Geometry check sheet. Reference: the model listing, model coordinates, mm. Face numbers are marked on the shaded views. Give positions to 0.01 mm unless a question says otherwise; leave off trailing zeros. Write each loop counter-clockwise with the first axis right and the second up, starting at its lowest first coordinate (ties: lowest second). Pieces come first, ordered by that corner, then holes. Notation, with made-up numbers: (72, 9) - (121, 9) arc R28 cw to (121, 40) - close; hole circle Ø7 at (59, 43). An arc over 180 degrees is marked (long way). One line per question, with ' | ' between items. Start each with the question number.
Q1. Section check A-A on x = -7.75. Record the boundary of the cut face in (y, z).
Q2. Thickness scan on L1, parallel to X at y = -0.35, z = 0.55; L2, parallel to X at y = 0.05, z = 0.85; L3, parallel to Y at x = -6.75, z = 0.8. Record the ranges inside material, lowest first. Write a range as [from, to].
Q3. Section check B-B on y = -2.25. Record the boundary of the cut face in (x, z).
Q4. Section check D-D on y = 0.6. Record the boundary of the cut face in (x, z).
Q5. Release check for a two-part mould opening along X. For the marked faces 1 and 2 record: +X half, -X half, draft (parallel to the pull), parting line (faces both ways), or undercut.
Q6. Section check C-C on z = 0.85. Record the boundary of the cut face in (x, y) (1 decimal), and give its area (3 significant figures).
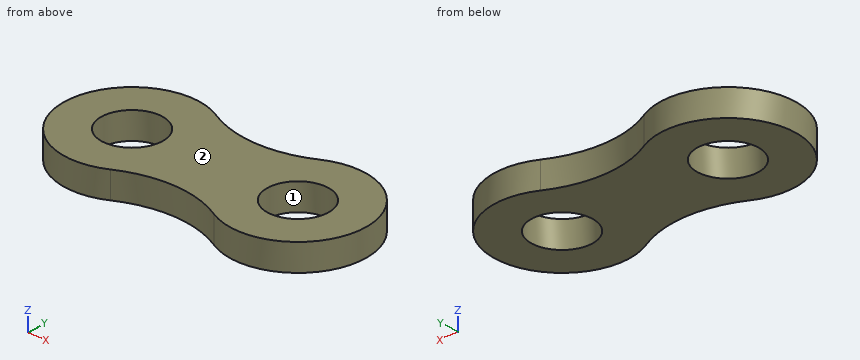
Autodesk Inventor part; units mm, degrees
ref_plane "YZ Plane" through (0, 0, 0) normal (1, 0, 0) x (0, 1, 0)
ref_plane "XZ Plane" through (0, 0, 0) normal (0, 1, 0) x (-1, 0, 0)
ref_plane "XY Plane" through (0, 0, 0) normal (0, 0, 1) x (1, 0, 0)
sketch "Sketch1" plane through (0, 0, 0) normal (0, 0, 1) x (1, 0, 0)
  arc A0 (-11.9712, 1.9221) -> (-8.0178, 1.9221) centre (-9.9945, 5.5697) ccw
  arc A1 (-8.0178, -2.5002) -> (-8.0178, 1.9221) centre (-6.8195, -0.289) ccw
  arc A2 (-8.0178, -2.5002) -> (-11.9712, -2.5002) centre (-9.9945, -6.1478) ccw
  arc A3 (-11.9712, 1.9221) -> (-11.9712, -2.5002) centre (-13.1695, -0.289) ccw
  circle A4 centre (-13.1695, -0.289) radius 1.135
  circle A5 centre (-6.8195, -0.289) radius 1.135
  point P0 (0, 0)
extrude "Extrusion1" add sketch "Sketch1" along normal blind 0.9906
properties part number "Chain Link"
Working result:
1) outline: (-2.63, 0) - (-0.94, 0) - (-0.94, 0.99) - (-2.63, 0.99) - close; (0.36, 0) - (2.05, 0) - (2.05, 0.99) - (0.36, 0.99) - close
2) L1: x = [-15.68, -14.3], [-12.04, -7.95], [-5.69, -4.31] | L2: x = [-15.66, -14.25], [-12.09, -7.9], [-5.74, -4.33] | L3: y = [-2.8, -1.42], [0.84, 2.22]
3) outline: (-14.74, 0) - (-11.42, 0) - (-11.42, 0.99) - (-14.74, 0.99) - close; (-8.57, 0) - (-5.24, 0) - (-5.24, 0.99) - (-8.57, 0.99) - close
4) outline: (-15.52, 0) - (-13.88, 0) - (-13.88, 0.99) - (-15.52, 0.99) - close; (-12.46, 0) - (-7.53, 0) - (-7.53, 0.99) - (-12.46, 0.99) - close; (-6.11, 0) - (-4.47, 0) - (-4.47, 0.99) - (-6.11, 0.99) - close
5) face 1: undercut | face 2: draft
6) outline: (-12, -2.5) arc R4.1 cw to (-8, -2.5) arc R2.5 ccw (long way) to (-8, 1.9) arc R4.1 cw to (-12, 1.9) arc R2.5 ccw (long way) to start; hole circle Ø2.3 at (-13.2, -0.3); hole circle Ø2.3 at (-6.8, -0.3) | area: 38.2 mm2
